Autodesk Inventor part; units mm, degrees
ref_plane "YZ Plane" through (0, 0, 0) normal (1, 0, 0) x (0, 1, 0)
ref_plane "XZ Plane" through (0, 0, 0) normal (0, 1, 0) x (-1, 0, 0)
ref_plane "XY Plane" through (0, 0, 0) normal (0, 0, 1) x (1, 0, 0)
sketch "スケッチ1" plane through (0, 0, 0) normal (0, 0, 1) x (1, 0, 0)
  line L0 (0, 0) -> (40, 0)
  line L1 (40, 0) -> (40, 318)
  line L2 (40, 318) -> (0, 318)
  line L3 (0, 318) -> (0, 0)
  line L4 (0, 218) -> (112.7627, 152.8964)
  line L5 (112.7627, 152.8964) -> (132.7627, 187.5375)
  line L6 (132.7627, 187.5375) -> (40, 241.094)
  point P0 (40, 218)
  point P1 (40, 194.906)
  point P2 (20, 318)
  point P3 (122.7627, 170.2169)
  point P4 (20, 258)
  dimension "d0" = 40
  dimension "d1" = 318
  dimension "d69" = 40
  dimension "d70" = 60
  dimension "d91" = 20
  dimension "d92" = 100
  dimension "d93" = 180
  dimension "d96" = 20
  dimension "d97" = 60
extrude "押し出し1" add sketch "スケッチ1" along normal blind 19.6 contours L3 L2 L1 L4 | L1 L6 L5 L4
sketch "スケッチ6" plane through (0, 0, 19.6) normal (0, 0, 1) x (1, 0, 0)
  circle A0 centre (20, 268) radius 7
  line L0 (40, 318) -> (0, 318)
  line L1 (40, 241.094) -> (40, 318)
  circle A1 centre (20, 20) radius 1.2295
  circle A2 centre (20, 10) radius 1.2295
  line L2 (0, 0) -> (40, 0)
  circle A3 centre (20, 298) radius 4
  point P0 (20, 318)
  point P1 (40, 190.8114)
  point P2 (30, 0)
  dimension "d42" = 14
  dimension "d44" = 20
  dimension "d45" = 2.459
  dimension "d46" = 2.459
  dimension "d47" = 10
  dimension "d48" = 10
  dimension "d49" = 20
  dimension "d50" = 20
  dimension "d53" = 8
  dimension "d54" = 20
  dimension "d55" = 30
  dimension "d56" = 20
extrude "押し出し4" cut sketch "スケッチ6" against normal through all contours A0 | A3
sketch "スケッチ8" plane through (0, 0, 0) normal (-1, 0, 0) x (0, 0, 1)
  line L0 (0, 318) -> (19.6, 318)
  line L1 (5, 318) -> (14.6, 318)
  line L2 (14.6, 318) -> (14.6, 278)
  line L3 (14.6, 278) -> (5, 278)
  line L4 (5, 278) -> (5, 318)
  line L5 (0, 318) -> (0, 0)
  dimension "d57" = 5
  dimension "d58" = 9.6
  dimension "d59" = 40
  dimension "d98" = 19.6
extrude "押し出し5" cut sketch "スケッチ8" against normal through all
fillet "フィレット1" radius 20 4 edges at (40, 318, 17.1) (40, 318, 2.5) (0, 318, 2.5) (0, 318, 17.1)
fillet "フィレット2" radius 40 2 edges at (0, 218, 9.8) (40, 241.094, 9.8)
sketch "スケッチ9" plane through (0, 0, 19.6) normal (0, 0, 1) x (1, 0, 0)
  line L0 (20, 206.453) -> (112.7627, 152.8964)
  line L1 (132.7627, 187.5375) -> (60, 229.547)
  line L2 (112.7627, 152.8964) -> (132.7627, 187.5375)
  line L3 (132.7627, 187.5375) -> (112.7627, 152.8964)
  line L4 (66.3813, 179.6747) -> (112.7627, 152.8964)
  line L5 (132.7627, 187.5375) -> (166.773, 167.9016)
  line L6 (115.1204, 126.9801) -> (133.5174, 158.8446)
  line L7 (141.7531, 173.1092) -> (128.7627, 180.6092)
  line L8 (112.7627, 152.8964) -> (20, 206.453)
  line L9 (132.7627, 187.5375) -> (60, 229.547)
  line L10 (115.1204, 126.9801) -> (125.7531, 145.3964)
  line L11 (133.5174, 158.8446) -> (145.7531, 180.0375)
  line L12 (116.7627, 159.8246) -> (129.7531, 152.3246)
  line L13 (66.3813, 179.6747) -> (129.7531, 152.3246)
  line L14 (66.3813, 179.6747) -> (86.3813, 214.3157)
  line L15 (86.3813, 214.3157) -> (141.7531, 173.1092)
  point P0 (0, 0)
  point P1 (254.4532, 80.329)
  point P2 (128.7627, 180.6092)
  point P3 (123.2579, 156.0746)
  point P4 (86.3813, 214.3157)
  point P5 (40, 194.906)
  point P6 (115.8875, 158.3088)
  point P7 (129.6379, 182.1251)
  dimension "d80" = 24
  dimension "d81" = 40
  dimension "d83" = 15
  dimension "d84" = 8
  dimension "d90" = 24
extrude "押し出し6" cut sketch "スケッチ9" against normal through all contours L13 L2 L0 | L1 L2 L15
sketch "スケッチ11" plane through (104.9897, 139.4332, 24) normal (0.8660254, -0.5, 0) x (0, 0, -1)
  line L0 (4.4, 21.7957) -> (4.4, 49.2964)
  line L1 (24, 21.7957) -> (24, 49.2964)
  line L2 (0, 24) -> (24, 24)
  line L3 (24, 24) -> (24, 0)
  line L4 (24, 0) -> (0, 0)
  line L5 (0, 0) -> (0, 24)
  line L6 (17, 17) -> (7, 17)
  line L7 (7, 17) -> (7, 7)
  line L8 (7, 7) -> (17, 7)
  line L9 (17, 7) -> (17, 17)
  line L10 (4.4, 35.546) -> (24, 35.546)
  circle A0 centre (14.2, 35.546) radius 5
  point P0 (24, -173.2475)
  point P1 (24, 24)
  point P2 (0, 15.546)
  point P3 (24, 15.546)
  dimension "d85" = 10
  dimension "d88" = 10
extrude "押し出し7" add sketch "スケッチ11" along normal blind 15 contours A0 L10 | L10 A0
fillet "フィレット4" radius 20 2 edges at (0, 278, 9.8) (40, 278, 9.8)
sketch "スケッチ12" plane through (0, 0, 19.6) normal (0, 0, 1) x (1, 0, 0)
  line L0 (0, 340.2847) -> (40, 340.2847)
  line L1 (40, 340.2847) -> (40, 181.2581)
  line L2 (40, 181.2581) -> (0, 181.2581)
  line L3 (0, 181.2581) -> (0, 340.2847)
  line L4 (40, 264.188) -> (40, 298)
  arc A0 (40, 298) -> (0, 298) centre (20, 298) ccw
  arc A1 (40, 264.188) -> (60, 229.547) centre (80, 264.188) ccw
  line L5 (60, 229.547) -> (40, 194.906)
  line L6 (20, 206.453) -> (66.3813, 179.6747)
  arc A2 (0, 241.094) -> (20, 206.453) centre (40, 241.094) ccw
  arc A3 (0, 241.094) -> (20, 206.453) centre (40, 241.094) ccw
  line L7 (20, 206.453) -> (40, 194.906)
  line L8 (86.3813, 214.3157) -> (60, 229.547)
  line L9 (60, 229.547) -> (86.3813, 214.3157)
  line L10 (86.3813, 214.3157) -> (66.3813, 179.6747)
  line L11 (40, 194.906) -> (66.3813, 179.6747)
  circle A4 centre (20, 298) radius 4
  circle A5 centre (20, 268) radius 7
  circle A6 centre (20, 268) radius 4
  point P0 (0, 0)
  dimension "d99" = 40
  dimension "d100" = 40
extrude "押し出し8" add sketch "スケッチ12" along normal blind 5 contours A0 L1 L6 A2 L3 | A1 L5 L1 | L5 L8 L10 L6
sketch "スケッチ13" plane through (0, 0, 0) normal (0, 0, -1) x (-1, 0, 0)
  line L0 (-253.843, 397.4333) -> (123.9074, 397.4333)
  line L1 (123.9074, 397.4333) -> (123.9074, 95.9261)
  line L2 (123.9074, 95.9261) -> (-253.843, 95.9261)
  line L3 (-253.843, 95.9261) -> (-253.843, 397.4333)
  point P0 (0, 0)
extrude "押し出し9" cut sketch "スケッチ13" against normal blind 19.6
sketch "スケッチ14" plane through (0, 0, 24.6) normal (0, 0, 1) x (1, 0, 0)
  line L0 (20, 206.453) -> (66.3813, 179.6747)
  line L1 (66.3813, 179.6747) -> (86.3813, 214.3157)
  line L2 (41.7403, 216.9952) -> (76.3813, 196.9952)
  point P0 (0, 0)
  point P1 (67.7211, 201.9952)
  dimension "d105" = 20
  dimension "d106" = 20
  dimension "d107" = 30
  dimension "d108" = 10
hole "穴3" at (41.7403, 216.9952, 24.6) at (67.7211, 201.9952, 24.6) direction (0, 0, -1) diameter 3 end through all
fillet "フィレット5" radius 5 2 edges at (86.3813, 214.3157, 22.1) (66.3813, 179.6747, 22.1)
sketch "スケッチ16" plane through (0, 0, 19.6) normal (0, 0, -1) x (-1, 0, 0)
  circle A0 centre (-67.7211, 201.9952) radius 1.5
  circle A1 centre (-67.7211, 201.9952) radius 3
  circle A2 centre (-41.7403, 216.9952) radius 1.5
  circle A3 centre (-41.7403, 216.9952) radius 3
  point P0 (0, 0)
  dimension "d121" = 6
  dimension "d122" = 6
extrude "押し出し11" cut sketch "スケッチ16" against normal blind 3 contours A0 | A1 | A2 | A3
sketch "スケッチ17" plane through (0, 0, 19.6) normal (0, 0, -1) x (-1, 0, 0)
  circle A0 centre (-20, 298) radius 4
  circle A1 centre (-20, 298) radius 6.5
  line L0 (-25, 306.9818) -> (-15, 306.9818)
  line L1 (-15, 306.9818) -> (-15, 289.1648)
  line L2 (-15, 289.1648) -> (-25, 289.1648)
  line L3 (-25, 289.1648) -> (-25, 306.9818)
  point P0 (0, 0)
  point P1 (-25, 302.1533)
  point P2 (-25, 293.8467)
  point P3 (-15, 293.8467)
  point P4 (-15, 302.1533)
  dimension "d125" = 13
  dimension "d126" = 5
  dimension "d127" = 10
extrude "押し出し12" cut sketch "スケッチ17" against normal blind 2 contours L1 A1 L3
equation "\"d45\" = d46"
equation "\"d48\" = d47"
equation "\"d50\" = d49"
equation "\"d106\" = d105"
properties part number "BR_parts_06(3)" material "アルミニウム 6061"
Here's how the part is built. I have some questions about the finished solid (model axes, mm). A direction names the side the tool comes from. Give positions to 0.01 mm unless a question says otherwise; leave off trailing zeros. Write each loop counter-clockwise with the first axis right and the second up, starting at its lowest first coordinate (ties: lowest second). Pieces come first, ordered by that corner, then holes. Notation, with made-up numbers: M -5,72.25 L 34,72.25 A18 ccw 34,91.25 Z; hole C 33.25,27.5 d5. An arc over 180 degrees is marked long. Put each result on its own line as item: value. Start each with the question number.
Item 1: I need wall thicknesses on L1, parallel to Y at x = 20, z = 23; L2, parallel to Y at x = 24, z = 20.2; L3, parallel to X at y = 268, z = 21. Which ranges of each line are inside material? Lowest first, please. Write a range as from..to.
Item 2: Thinking about a two-plate mould opening in X: for faces 1 (the flat face through (20.1, 293.8, 21.6)), 2 (the flat face through (40, 281, 22)), 3 (the flat face through (0, 270, 22)), which applies, +X half, -X half, draft (parallel to the pull), parting line (faces both ways), or undercut?
Item 3: On a 3-axis mill with a long thin cutter (end or side, diameter ignored), from which of +Z, -Z, +X, -X, +Y, -Y can I reach the whole of each face in a straight line? I mean faces 4 (the cylindrical face through (18.483, 274.834, 22.065)), 5 (the flat face through (66, 201, 22.6)). Say none if no direction works.
Item 4: If we section it at B-B, the plane z = 23.55: Write out the boundary of the cut face in (x, y), then the cut area to 3 significant figures.
Item 5: If we section it at A-A, the plane y = 268: Write out the boundary of the cut face in (x, z), then the cut area to 3 significant figures.
Item 6: If we section it at C-C, the plane x = 35.5: Write out the boundary of the cut face in (y, z).
Item 7: Will these pins go through, and if not, where does the flat tip stop? pin 1 (4 mm diameter, centred on x = 41.74, y = 217, fed in from +Z); pin 2 (5 mm diameter, centred on x = 67.72, y = 202, fed in from -Z); pin 3 (5 mm diameter, centred on x = 63.5, y = 230.5, fed in from +Z); pin 4 (3 mm diameter, centred on x = 61.5, z = 21.5, fed in from +Y).
Item 8: If we section it at D-D, the plane y = 193.5: Write out the boundary of the cut face in (x, z).
Values:
1. L1: 206.45..261, 275..294, 302..318
1. L2: 204.14..262.26, 273.74..292.88, 303.12..317.6
1. L3: 0..13, 27..40
2. face 1: undercut
2. face 2: +X half
2. face 3: -X half
3. face 4: +Z, -Z
3. face 5: -Z
4. outline: M 0,241.09 A40 ccw 20,206.45 L 62.05,182.17 A5 ccw 68.88,184 L 83.88,209.99 A5 ccw 82.05,216.82 L 60,229.55 A40 cw 40,264.19 L 40,298 A20 ccw 0,298 Z; hole C 20,268 d14; hole C 20,298 d8; hole C 41.74,217 d3; hole C 67.72,202 d3
4. area: 5,740 mm²
5. outline: M 0,19.6 L 13,19.6 L 13,24.6 L 0,24.6 Z; M 27,19.6 L 40,19.6 L 40,24.6 L 27,24.6 Z
5. area: 130 mm²
6. outline: M 197.5,19.6 L 310.64,19.6 L 310.64,24.6 L 197.5,24.6 Z
7. pin 1: z = 24.6
7. pin 2: z = 22.6
7. pin 3: through
7. pin 4: y = 229.55
8. outline: M 42.44,19.6 L 74.36,19.6 L 74.36,24.6 L 42.44,24.6 Z
